Check sheet for the modelled part. Datum: model origin and axes. Units: mm. Give positions to 0.01 mm unless a question says otherwise; leave off trailing zeros. Order: outer loops, then holes, each group sorted by start corner. A loop starts at its lowest first (then second) coordinate and runs counter-clockwise, first axis right, second up. Notation, with made-up numbers: (-37, 88) - (-22, 88) arc R7 ccw to (-22, 99) - close; hole circle Ø3 at (-38.75, 36.25). An arc over 180 degrees is marked (long way). Answer in a Markdown table with one row per item.
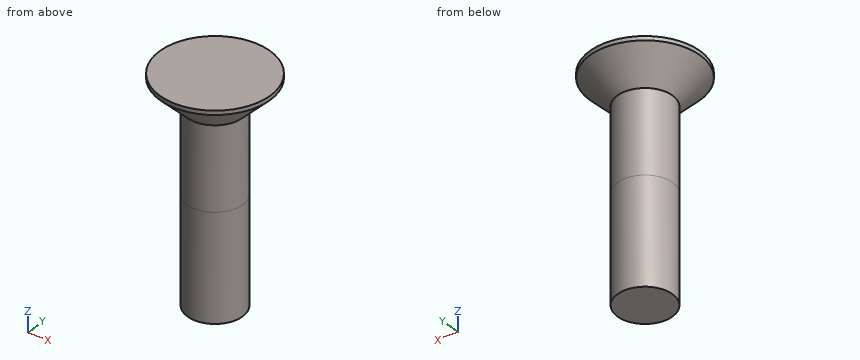
Autodesk Inventor part; units mm, degrees
ref_plane "YZ Plane" through (0, 0, 0) normal (1, 0, 0) x (0, 1, 0)
ref_plane "XZ Plane" through (0, 0, 0) normal (0, 1, 0) x (-1, 0, 0)
ref_plane "XY Plane" through (0, 0, 0) normal (0, 0, 1) x (1, 0, 0)
sketch "スケッチ1" plane through (0, 0, 0) normal (0, 0, 1) x (1, 0, 0)
  circle A0 centre (0, 0) radius 2
  dimension "d0" = 4
extrude "押し出し1" add sketch "スケッチ1" along normal blind 6
sketch "スケッチ2" plane through (0, 0, 6) normal (0, 0, 1) x (1, 0, 0)
  circle A0 centre (0, 0) radius 2
  circle A1 centre (0, 0) radius 4
  dimension "d3" = 8
extrude "押し出し2" add sketch "スケッチ2" along normal blind 2.3 contours A0 | A1
thread "ねじ1"
chamfer "面取り1" distance 2 angle 45 1 edges at (-4, 0, 6)
sketch "スケッチ4" plane through (0, 0, 0) normal (0, 0, -1) x (-1, 0, 0)
  circle A0 centre (0, 0) radius 2
extrude "押し出し4" add sketch "スケッチ4" along normal blind 7.7
properties part number "SB　M4 16mm 皿ネジ" material "Stainless Steel, 440C"
(1) Gauge pin test, flat ends, axial feed: P1, Ø1, axis at x = 1, z = 4, coming from the -Y side; P2, Ø2, axis at y = 1.5, z = 3, coming from the -X side; P3, Ø2, axis at y = -2.5, z = 3, coming from the +X side. Record the tip position at first contact, or that the pin passes through.
Geometry says:
| item | result |
|---|---|
| P1 | y = -1.94 |
| P2 | x = -1.94 |
| P3 | x = 1.32 |
(2) Cross-section at C-C, the plane z = -1.25. Record the cut outline in (x, y), then the cut area to 3 significant figures.
Geometry says:
| item | result |
|---|---|
| outline | circle Ø4 at (0, 0) |
| area | 12.6 mm² |
(3) Cross-section at D-D, the plane z = 7.5. Record the cut outline in (x, y).
Geometry says:
| item | result |
|---|---|
| outline | circle Ø7 at (0, 0) |
(4) Thickness scan on L1, parallel to X at y = 0, z = 6.5; L2, parallel to Y at x = 0, z = -6.25; L3, parallel to X at y = -0.25, z = 1.5. Record the ranges inside material, lowest first.
Geometry says:
| item | result |
|---|---|
| L1 | -2.5 to 2.5 |
| L2 | -2 to 2 |
| L3 | -1.98 to 1.98 |
